from build123d import *

# Parameters (mm, degrees)
RESSALTO_EXTRUS_O1_DEPTH = 10
ESBO_O2_R                = 2.5
CORTE_EXTRUS_O1_DEPTH    = 10
FILETE1_R                = 5
CORTE_EXTRUS_O4_DEPTH    = 10
CORTE_EXTRUS_O5_DEPTH    = 10
CORTE_EXTRUS_O6_REACH    = 39.417
ESBO_O7_W                = 15
ESBO_O7_H                = 10
ESBO_O8_W                = 11
ESBO_O8_H                = 10
CORTE_EXTRUS_O7_DEPTH    = 27.925824036
CORTE_EXTRUS_O8_DEPTH    = 20
CORTE_EXTRUS_O9_REACH    = 39.417
ESBO_O10_R               = 2.5
FILETE2_R                = 5


with BuildPart() as part:
    # Esboço1 → Ressalto-extrusão1 (new body)
    with BuildSketch(Plane.XY):
        Polygon((-10, -7.5), (20, 15), (-10, 15), (-10, 4.8), (-20, 4.8), (-20, -4.8), (-10, -4.8), align=None)
        Polygon((20, -15), (20, 15), (-10, -7.5), (-10, -15), align=None)
    extrude(amount=RESSALTO_EXTRUS_O1_DEPTH)

    # Esboço2 → Corte-extrusão1 (cut)
    with BuildSketch(Plane.XZ.offset(4.8)):
        with Locations(Location((-15, 5, 0), (0, 0, 270))):
            Circle(ESBO_O2_R)
    extrude(amount=-CORTE_EXTRUS_O1_DEPTH, mode=Mode.SUBTRACT)

    # Filete1
    filete1_edges = [part.edges().sort_by_distance(p)[0] for p in [
        (-20, 0, 0),
        (-20, 0, 10),
    ]]
    fillet(filete1_edges, radius=FILETE1_R - 0.0001)  # a hair under: the kernel refuses the full size

    # Esboço5 → Corte-extrusão4 (cut)
    with BuildSketch(Plane.XZ.offset(15)):
        with BuildLine():
            Line((-10, 10), (-10, 0))
            ThreePointArc((-10, 0), (-9.341737512, 5), (-10, 10))
        make_face()
    extrude(amount=-CORTE_EXTRUS_O4_DEPTH, mode=Mode.SUBTRACT)

    # Esboço6 → Corte-extrusão5 (cut)
    with BuildSketch(Plane(origin=(0, 15, 0), x_dir=(1, 0, 0), z_dir=(0, 1, 0))):
        with BuildLine():
            Line((-10, -9.950546275), (-10, 0))
            ThreePointArc((-10, 0), (-9.344992865, -4.975273137), (-10, -9.950546275))
        make_face()
    extrude(amount=-CORTE_EXTRUS_O5_DEPTH, mode=Mode.SUBTRACT)

    # Esboço7 → Corte-extrusão6 (cut, up to next)
    with BuildSketch(Plane(origin=(0, 15, 0), x_dir=(1, 0, 0), z_dir=(0, 1, 0)), mode=Mode.PRIVATE) as corte_extrus_o6_sk1:
        with Locations((12.5, -5)):
            Rectangle(ESBO_O7_W, ESBO_O7_H)
    corte_extrus_o6_tool1 = extrude(corte_extrus_o6_sk1.sketch, amount=-CORTE_EXTRUS_O6_REACH, mode=Mode.PRIVATE) & part.part
    add(corte_extrus_o6_tool1.solids().sort_by_distance((12.5, 15, 5))[0], mode=Mode.SUBTRACT)

    # Esboço8 → Corte-extrusão7 (cut, through all)
    with BuildSketch(Plane.XY.offset(10)):
        with Locations((-0.5, 0)):
            Rectangle(ESBO_O8_W, ESBO_O8_H)
    extrude(amount=-CORTE_EXTRUS_O7_DEPTH, mode=Mode.SUBTRACT)

    # Esboço9 → Corte-extrusão8 (cut)
    with BuildSketch(Plane(origin=(0, 0, 0), x_dir=(-1, 0, 0), z_dir=(0, 0, -1))):
        with BuildLine():
            Line((6, -5), (6, 5))
            ThreePointArc((6, 5), (6.419601085, 0), (6, -5))
        make_face()
    extrude(amount=-CORTE_EXTRUS_O8_DEPTH, mode=Mode.SUBTRACT)

    # Corte-extrusão9: up to this face of the body (flat: up to its plane)
    corte_extrus_o9_end = Plane(part.part.faces().sort_by_distance((-2.281136508, -15, 5))[0])
    # Esboço10 → Corte-extrusão9 (cut, up to the picked face)
    with BuildSketch(Plane(origin=(0, 15, 0), x_dir=(1, 0, 0), z_dir=(0, 1, 0)), mode=Mode.PRIVATE) as corte_extrus_o9_sk1:
        with Locations(Location((0, -5, 0), (0, 0, 180))):
            Circle(ESBO_O10_R)
    corte_extrus_o9_tool1 = split(extrude(corte_extrus_o9_sk1.sketch, amount=-CORTE_EXTRUS_O9_REACH, mode=Mode.PRIVATE), bisect_by=corte_extrus_o9_end, keep=Keep.BOTH, mode=Mode.PRIVATE)
    add(corte_extrus_o9_tool1.solids().sort_by(Axis((0, 15, 5), (0, -1, 0)))[0], mode=Mode.SUBTRACT)

    # Filete2
    filete2_edges = [part.edges().sort_by_distance(p)[0] for p in [
        (5, -10, 0),
        (5, -10, 10),
        (5, 10, 10),
        (5, 10, 0),
    ]]
    fillet(filete2_edges, radius=FILETE2_R - 0.0001)  # a hair under: the kernel refuses the full size


solid = part.part
Geometry: final body of the model. Coordinates: model frame, mm. A direction names the side the tool comes from. Give positions to 0.01 mm unless a question says otherwise; leave off trailing zeros. Order: outer loops, then holes, each group sorted by start corner. A loop starts at its lowest first (then second) coordinate and runs counter-clockwise, first axis right, second up. Notation, with made-up numbers: (32, 77.25) - (74, 77.25) arc R23 cw to (74, 91.25) - close; hole circle Ø5 at (-26, 26). An arc over 180 degrees is marked (long way). Use CSV: the item, a comma, the result in double quotes.
1. Mould query, pull axis X, two halves, no side actions, for faces 4 (the face through (-8, 0, 10)), 5 (the face through (-15.96, -0.07, 2.69)), 6 (the face through (-6.42, 0.07, 4.93)). Classes: +X half, -X half, draft (parallel to the pull), parting line (faces both ways), or undercut.
Answers below:
face 4,"draft"
face 5,"undercut"
face 6,"+X half"
2. Section query C-C (z = 8). Output: boundary loops of the cut face in (x, y), plus the area to 3 significant figures.
Answers below:
outline,"(-19, -4.8) - (-10, -4.8) - (-10, -5) - (-9.58, -5) - (-9.58, -15) - (4, -15) - (4, -5) - (-6, -5) arc R30 cw to (-6, 5) - (4, 5) - (4, 15) - (-9.58, 15) - (-9.58, 5) - (-10, 5) - (-10, 4.8) - (-19, 4.8) - close"
area,"395 mm2"
3. Material intervals for line 1 along Z through (x, y) = (0, 8.25); line 2 along Y through (x, z) = (-1.5, 2.25); line 3 along X through (y, z) = (-2, 3.25), sorted ascending. Write a range as from..to.
Answers below:
line 1,"0..2.5, 7.5..10"
line 2,"-15..-5, 5..15"
line 3,"-19.68..-16.79, -13.21..-6.35"
4. Access query for faces 1 (the face through (-3, -5, 5)), 2 (the face through (-9.345, 10.07, 4.905)), 3 (the face through (-13, 4.8, 3)). Directions: +Z, -Z, +X, -X, +Y, -Y. A direction counts if a zero-diameter tool reaches every point of the face in a straight line with its end or side. Return the directions, or none.
Answers below:
face 1,"+Z, -Z, +X"
face 2,"-X, +Y"
face 3,"+Z, -Z, -X, +Y"
5. Contact query for flat-ended pins moving along their axis: pin 1 (3 mm diameter, centred on y = 12, z = 3, fed in from -X); pin 2 (2 mm diameter, centred on y = 9.5, z = 1.5, fed in from -X); pin 3 (4 mm diameter, centred on y = 2.5, z = 8, fed in from +X). Output: stop coordinate, or through.
Answers below:
pin 1,"x = -9.66"
pin 2,"x = -9.87"
pin 3,"x = -6.08"
6. Section query A-A (x = -3.25). Output: boundary loops of the cut face in (y, z), plus the area to 3 significant figures.
Answers below:
outline,"(-15, 0) - (-5, 0) - (-5, 10) - (-15, 10) - close; (5, 0) - (15, 0) - (15, 10) - (5, 10) - close"
area,"200 mm2"
7. Section query D-D (z = 6.5). Output: boundary loops of the cut face in (x, y).
Answers below:
outline,"(-19.77, -4.8) - (-17, -4.8) - (-17, 4.8) - (-19.77, 4.8) - close; (-13, -4.8) - (-10, -4.8) - (-10, -5) - (-9.4, -5) - (-9.4, -15) - (-2, -15) - (-2, -5) - (-6, -5) arc R30 cw to (-6, 5) - (-2, 5) - (-2, 15) - (-9.41, 15) - (-9.41, 5) - (-10, 5) - (-10, 4.8) - (-13, 4.8) - close; (2, -15) - (4.77, -15) - (4.77, -5) - (2, -5) - close; (2, 5) - (4.77, 5) - (4.77, 15) - (2, 15) - close"
